Autodesk Inventor part; units mm, degrees
ref_plane "YZ Plane" through (0, 0, 0) normal (1, 0, 0) x (0, 1, 0)
ref_plane "XZ Plane" through (0, 0, 0) normal (0, 1, 0) x (-1, 0, 0)
ref_plane "XY Plane" through (0, 0, 0) normal (0, 0, 1) x (1, 0, 0)
sketch "Boceto1" plane through (0, 0, 0) normal (0, 1, 0) x (-1, 0, 0)
  line L0 (-9.525, 19.05) -> (9.525, 19.05)
  line L1 (9.525, 19.05) -> (9.525, -19.05)
  line L2 (9.525, -19.05) -> (-9.525, -19.05)
  line L3 (-9.525, -19.05) -> (-9.525, 19.05)
  line L4 (-9.525, 19.05) -> (9.525, -19.05) construction
  line L5 (9.525, 19.05) -> (-9.525, -19.05) construction
  point P0 (0, 0)
  dimension "d0" = 19.05
  dimension "d1" = 38.1
extrude "Extrusión1" add sketch "Boceto1" along normal blind 12.7
sketch "Boceto3" plane through (9.525, 0, 19.05) normal (1, 0, 0) x (0, 0, -1)
  line L0 (38.1, 0) -> (38.1, 12.7)
  line L1 (38.1, 6.35) -> (38.1, 6.35)
  line L2 (0, 6.35) -> (0, 6.35)
  arc A0 (6.35, 12.7) -> (0, 6.35) centre (6.35, 6.35) ccw
  arc A1 (0, 6.35) -> (6.35, 0) centre (6.35, 6.35) ccw
  arc A2 (38.1, 6.35) -> (31.75, 12.7) centre (31.75, 6.35) ccw
  arc A3 (31.75, 0) -> (38.1, 6.35) centre (31.75, 6.35) ccw
  line L3 (0, 0) -> (0, 12.7)
  line L4 (38.1, 0) -> (31.75, 0)
  line L5 (6.35, 0) -> (0, 0)
  line L6 (0, 12.7) -> (6.35, 12.7)
  line L7 (31.75, 12.7) -> (38.1, 12.7)
  point P0 (19.05, 0)
  point P1 (0, 6.35)
  dimension "d7" = 6.35
extrude "Extrusión3" cut sketch "Boceto3" against normal up to surface (19.05 mm away)
sketch "Boceto5" plane through (0, 12.7, 0) normal (0, 1, 0) x (1, 0, 0)
  line L0 (-9.525, 19.05) -> (-9.525, -19.05)
  line L1 (9.525, -12.7) -> (9.525, 12.7)
  line L2 (9.525, -19.05) -> (9.525, -12.7)
  line L3 (-8.025, -3.843) -> (-8.025, -19.05)
  line L4 (8.025, -3.843) -> (8.025, -12.7)
  line L5 (8.025, -12.7) -> (8.025, -19.05)
  line L6 (-8.025, -3.843) -> (8.025, -3.843)
  line L7 (-8.025, -19.05) -> (8.025, -19.05)
  line L8 (-9.525, -19.05) -> (9.525, -19.05)
  point P0 (0, 0)
  dimension "d11" = 1.5
  dimension "d12" = 1.5
extrude "Extrusión4" cut sketch "Boceto5" against normal up to surface (12.7 mm away)
sketch "Boceto6" plane through (9.525, 0, 12.7) normal (1, 0, 0) x (0, 0, -1)
  arc A0 (0, 12.7) -> (0, 0) centre (0, 6.35) ccw
  circle A1 centre (0, 6.35) radius 2.54
  point P0 (12.7, 0)
  dimension "d15" = 5.08
extrude "Extrusión5" cut sketch "Boceto6" against normal up to surface (19.05 mm away)
sketch "Boceto7" plane through (9.525, 0, 12.7) normal (1, 0, 0) x (0, 0, -1)
  line L0 (0, 12.7) -> (25.4, 12.7)
  arc A0 (16.5105, 12.7) -> (16.5105, 0) centre (27.5091, 6.35) ccw
  line L1 (16.5105, 12.7) -> (35.1863, 12.7)
  line L2 (35.1863, 12.7) -> (35.1863, 0)
  line L3 (35.1863, 0) -> (16.5105, 0)
  circle A1 centre (25.4, 6.35) radius 2.54
  point P0 (12.7, 0)
  dimension "d18" = 12.7
  dimension "d19" = 5.08
extrude "Extrusión6" cut sketch "Boceto7" against normal blind 1.5
sketch "Boceto8" plane through (-9.525, 0, -12.7) normal (-1, 0, 0) x (0, 0, 1)
  arc A0 (8.8895, 0) -> (8.8895, 12.7) centre (-2.1091, 6.35) ccw
  line L0 (-6.35, 12.7) -> (31.75, 12.7)
  line L1 (0, 0) -> (25.4, 0)
  circle A1 centre (0, 6.35) radius 2.54
  line L2 (0, 0) -> (-7.3331, 0)
  line L3 (-7.3331, 0) -> (-7.3331, 12.7)
  line L4 (-7.3331, 12.7) -> (-6.35, 12.7)
  point P0 (12.7, 0)
extrude "Extrusión7" cut sketch "Boceto8" against normal blind 1.5
sketch "Boceto9" plane through (-8.025, 12.7, 3.843) normal (0, 0, 1) x (1, 0, 0)
  line L0 (16.05, -12.7) -> (0, -12.7)
  line L1 (16.05, 0) -> (16.05, -12.7)
  line L2 (0, 0) -> (16.05, 0)
  line L3 (0, 0) -> (0, -12.7)
  line L4 (14.55, -1.5) -> (14.55, -11.2)
  line L5 (14.55, -11.2) -> (1.5, -11.2)
  line L6 (1.5, -11.2) -> (1.5, -1.5)
  line L7 (1.5, -1.5) -> (14.55, -1.5)
  point P0 (8.025, -12.7)
  dimension "d24" = 1.5
extrude "Extrusión8" cut sketch "Boceto9" against normal blind 25 contours L4 L5 L6 L7
sketch "Boceto10" plane through (0, 12.7, 0) normal (0, 1, 0) x (1, 0, 0)
  line L0 (6.525, 16.7988) -> (-6.525, 16.7988)
  line L1 (6.525, 16.7988) -> (6.525, 3.7495)
  line L2 (6.525, -3.843) -> (6.525, 16.7988)
  line L3 (-6.525, -3.843) -> (-6.525, 16.7988)
  line L4 (-6.525, 3.7495) -> (-6.525, 16.7988)
  line L5 (-6.525, 16.7988) -> (6.525, 16.7988)
  line L6 (-6.525, 3.7495) -> (6.525, 3.7495)
  point P0 (0, 0)
extrude "Extrusión9" cut sketch "Boceto10" against normal up to surface (12.7 mm away)
sketch "Boceto12" plane through (-8.025, 12.7, 3.843) normal (0, 0, 1) x (1, 0, 0)
  line L0 (0, 0) -> (-1.5, 0)
  line L1 (16.05, 0) -> (16.05, -12.7)
  line L2 (0, 0) -> (16.05, 0)
  line L3 (16.05, 0) -> (16.05, -1)
  line L4 (16.05, -1) -> (0, -1)
  line L5 (0, -1) -> (0, 0)
  line L6 (16.05, -12.7) -> (0, -12.7)
  line L7 (0, -12.7) -> (16.05, -12.7)
  line L8 (16.05, -12.7) -> (16.05, -11.7)
  line L9 (16.05, -11.7) -> (0, -11.7)
  line L10 (0, -11.7) -> (0, -12.7)
  point P0 (8.025, -12.7)
  dimension "d29" = 1
  dimension "d30" = 1
extrude "Extrusión10" add sketch "Boceto12" along normal blind 9
sketch "Boceto13" plane through (8.025, 0, 12.7) normal (1, 0, 0) x (0, 0, -1)
  line L0 (16.5105, 12.7) -> (25.4, 12.7)
  line L1 (23.5239, 12.7) -> (24.1756, 12.1558)
  line L2 (24.1756, 12.1558) -> (25.9001, 12.2114)
  line L3 (25.9001, 12.2114) -> (30.8267, 9.6476)
  arc A0 (25.4, 0) -> (25.4, 12.7) centre (25.4, 6.35) ccw
  line L4 (23.5239, 12.7) -> (30.4855, 12.7)
  line L5 (30.4855, 12.7) -> (30.8267, 9.6476)
  point P0 (12.7, 0)
extrude "Extrusión11" cut sketch "Boceto13" against normal up to surface (16.05 mm away)
sketch "Boceto14" plane through (6.525, 12.7, -3.7495) normal (0, 0, -1) x (-1, 0, 0)
  line L0 (0, 0) -> (0, -1.5)
  line L1 (13.05, 0) -> (13.05, -1.5)
  line L2 (0, 0) -> (13.05, 0)
  line L3 (13.05, 0) -> (13.05, -1)
  line L4 (13.05, -1) -> (0, -1)
  line L5 (0, -1) -> (0, 0)
  line L6 (0, -11.2) -> (0, -12.7)
  line L7 (13.05, -11.2) -> (13.05, -12.7)
  line L8 (0, -12.7) -> (13.05, -12.7)
  line L9 (13.05, -12.7) -> (13.05, -11.7)
  line L10 (13.05, -11.7) -> (0, -11.7)
  line L11 (0, -11.7) -> (0, -12.7)
  point P0 (6.525, -12.7)
  point P1 (0, -1)
  dimension "d35" = 1
  dimension "d36" = 1
extrude "Extrusión12" add sketch "Boceto14" along normal blind 6
properties part number "cadena_link" material "Plástico PC/ABS"
Geometry: final body of the model. Coordinates: model frame, mm. A direction names the side the tool comes from. Round coordinates to 2 decimals unless told otherwise and drop trailing zeros. Order: outer loops, then holes, each group sorted by start corner. A loop starts at its lowest first (then second) coordinate and runs counter-clockwise, first axis right, second up. Notation, with made-up numbers: (63, 26) -> (75, 26) arc R10 cw to (75, 37) -> close; hole circle Ø7 at (22, 37). An arc over 180 degrees is marked (long way). Put each result on its own line as item: value. Start each with the question number.
Q1. First-contact query: pin 1 (4 mm diameter, centred on y = 3, z = -13.5, fed in from -X) (3 decimals); pin 2 (1 mm diameter, centred on y = 10, z = -13.5, fed in from +X) (3 decimals); pin 3 (0.8 mm diameter, centred on x = -0.5, y = 12, fed in from -Z); pin 4 (1.5 mm diameter, centred on x = 6.5, y = 11.5, fed in from -Z). Flat tips, straight axial feed; report the tip coordinate or a pass-through.
Q2. Section A-A on y = 6.35. Give the number of separate pieces and of enclosed holes in the cut face, and give its area (3 significant figures).
Q3. Pull-direction query (Y, two-part tool) for faces 5 (the flat face through (0, 11.2, 0)), 6 (the flat face through (7.286, 10.947, -15.629)), 7 (the flat face through (0.1, 0.5, -9.75)); classes: +Y half, -Y half, draft (parallel to the pull), parting line (faces both ways), or undercut.
Q4. Section C-C on x = 3.5. Return the cut outline in (y, z).
Q5. Reachability of faces 1 (the flat face through (-8.025, 6, 10)), 2 (the cylindrical face through (8.79, 8.87, -12.37)), 3 (the flat face through (0, 12, 12.843)), 4 (the flat face through (0, 1.5, 0)) from +Z, -Z, +X, -X, +Y, -Y: full face, straight path, thin tool, end or side. Return the list, or none.
Q6. Line query: probe 1 along Y at (x, z) = (3.5, 6); probe 2 along X at (y, z) = (6, -3.5) (3 decimals); probe 3 along X at (y, z) = (7.5, 16.5) (3 decimals). Output: solid intervals per line, ascending.
Q7. Section B-B on z = -5. Return the cut outline in (x, y) (3 decimals), and give its area (3 significant figures).
Q8. Section D-D on z = -16. Return the cut outline in (x, y) (3 decimals).
Ans:
1. pin 1: stops at x = -9.525
1. pin 2: stops at x = 8.025
1. pin 3: stops at z = -9.75
1. pin 4: stops at z = -16.01
2. separate pieces: 4
2. enclosed holes: 0
2. area: 132 mm2
3. face 5: undercut
3. face 6: +Y half
3. face 7: draft
4. outline: (0, -9.75) -> (1, -9.75) -> (1, -3.75) -> (1.5, -3.75) -> (1.5, 3.84) -> (1, 3.84) -> (1, 12.84) -> (0, 12.84) -> close; (11.2, -3.75) -> (11.7, -3.75) -> (11.7, -9.75) -> (12.7, -9.75) -> (12.7, 12.84) -> (11.7, 12.84) -> (11.7, 3.84) -> (11.2, 3.84) -> close
5. face 1: +Z
5. face 2: +X
5. face 3: +Z, +Y, -Y
5. face 4: +Z, -Z
6. probe 1: y = 0 to 1, 11.7 to 12.7
6. probe 2: x = -8.025 to -6.525, 6.525 to 8.025
6. probe 3: x = -9.525 to -8.025, 8.025 to 9.525
7. outline: (-8.025, 0) -> (8.025, 0) -> (8.025, 12.7) -> (-8.025, 12.7) -> close; hole (-6.525, 1) -> (6.525, 1) -> (6.525, 11.7) -> (-6.525, 11.7) -> close
7. area: 64.2 mm2
8. outline: (-8.025, 0.925) -> (-6.525, 0.925) -> (-6.525, 10.754) -> (-8.025, 10.754) -> close; (6.525, 0.925) -> (8.025, 0.925) -> (8.025, 10.754) -> (6.525, 10.754) -> close
